Geometry check sheet. Reference: the model listing, model coordinates, mm. Face numbers are marked on the shaded views. Give positions to 0.01 mm unless a question says otherwise; leave off trailing zeros. Write each loop counter-clockwise with the first axis right and the second up, starting at its lowest first coordinate (ties: lowest second). Pieces come first, ordered by that corner, then holes. Notation, with made-up numbers: (32.25, 34) -> (84.25, 34) arc R21 ccw to (84.25, 47) -> close; hole circle Ø1 at (-36, -3). An arc over 180 degrees is marked (long way). One line per item, written item: value.
from build123d import *

# Parameters (mm, degrees)
SKETCH1_W     = 490
SKETCH1_H     = 390
FRAME_DEPTH   = 40
OPENING_START = -1
SKETCH2_W     = 450
SKETCH2_H     = 350
OPENING_DEPTH = 42
PIVOT_0_START = -1
SKETCH3_R     = 3.3
PIVOT_0_DEPTH = 492
PIVOT_1_START = -1
SKETCH4_R     = 3.3
PIVOT_1_DEPTH = 492
PIVOT_2_START = -1
SKETCH5_R     = 3.3
PIVOT_2_DEPTH = 492
PIVOT_3_START = -1
SKETCH6_R     = 3.3
PIVOT_3_DEPTH = 492
PIVOT_4_START = -1
SKETCH7_R     = 3.3
PIVOT_4_DEPTH = 492
PIVOT_5_START = -1
SKETCH8_R     = 3.3
PIVOT_5_DEPTH = 492


with BuildPart() as part:
    # Sketch1 → frame (new body)
    with BuildSketch(Plane(origin=(0, 0, 0), x_dir=(0, 0, -1), z_dir=(1, 0, 0))):
        with Locations((-245, 195)):
            Rectangle(SKETCH1_W, SKETCH1_H)
    extrude(amount=FRAME_DEPTH)


with BuildPart() as body_2:
    # Sketch2 → opening (new body)
    with BuildSketch(Plane(origin=(0, 0, 0), x_dir=(0, 0, -1), z_dir=(1, 0, 0)).offset(OPENING_START)):
        with Locations((-245, 195)):
            Rectangle(SKETCH2_W, SKETCH2_H)
    extrude(amount=OPENING_DEPTH)


with BuildPart() as part_1:
    add(part.part)

    # Combine1: cut body 2
    add(body_2.part, mode=Mode.SUBTRACT)


with BuildPart() as body_2_2:
    # Sketch3 → pivot_0 (new body)
    with BuildSketch(Plane.XY.offset(PIVOT_0_START)):
        with Locations((20, 49.166666667)):
            Circle(SKETCH3_R)
    extrude(amount=PIVOT_0_DEPTH)


with BuildPart() as part_2:
    add(part_1.part)

    # Combine2: cut body 2 2
    add(body_2_2.part, mode=Mode.SUBTRACT)


with BuildPart() as body_2_3:
    # Sketch4 → pivot_1 (new body)
    with BuildSketch(Plane.XY.offset(PIVOT_1_START)):
        with Locations((20, 107.5)):
            Circle(SKETCH4_R)
    extrude(amount=PIVOT_1_DEPTH)


with BuildPart() as part_3:
    add(part_2.part)

    # Combine3: cut body 2 3
    add(body_2_3.part, mode=Mode.SUBTRACT)


with BuildPart() as body_2_4:
    # Sketch5 → pivot_2 (new body)
    with BuildSketch(Plane.XY.offset(PIVOT_2_START)):
        with Locations((20, 165.833333333)):
            Circle(SKETCH5_R)
    extrude(amount=PIVOT_2_DEPTH)


with BuildPart() as part_4:
    add(part_3.part)

    # Combine4: cut body 2 4
    add(body_2_4.part, mode=Mode.SUBTRACT)


with BuildPart() as body_2_5:
    # Sketch6 → pivot_3 (new body)
    with BuildSketch(Plane.XY.offset(PIVOT_3_START)):
        with Locations((20, 224.166666667)):
            Circle(SKETCH6_R)
    extrude(amount=PIVOT_3_DEPTH)


with BuildPart() as part_5:
    add(part_4.part)

    # Combine5: cut body 2 5
    add(body_2_5.part, mode=Mode.SUBTRACT)


with BuildPart() as body_2_6:
    # Sketch7 → pivot_4 (new body)
    with BuildSketch(Plane.XY.offset(PIVOT_4_START)):
        with Locations((20, 282.5)):
            Circle(SKETCH7_R)
    extrude(amount=PIVOT_4_DEPTH)


with BuildPart() as part_6:
    add(part_5.part)

    # Combine6: cut body 2 6
    add(body_2_6.part, mode=Mode.SUBTRACT)


with BuildPart() as body_2_7:
    # Sketch8 → pivot_5 (new body)
    with BuildSketch(Plane.XY.offset(PIVOT_5_START)):
        with Locations((20, 340.833333333)):
            Circle(SKETCH8_R)
    extrude(amount=PIVOT_5_DEPTH)


with BuildPart() as part_7:
    add(part_6.part)

    # Combine7: cut body 2 7
    add(body_2_7.part, mode=Mode.SUBTRACT)


solid = part_7.part
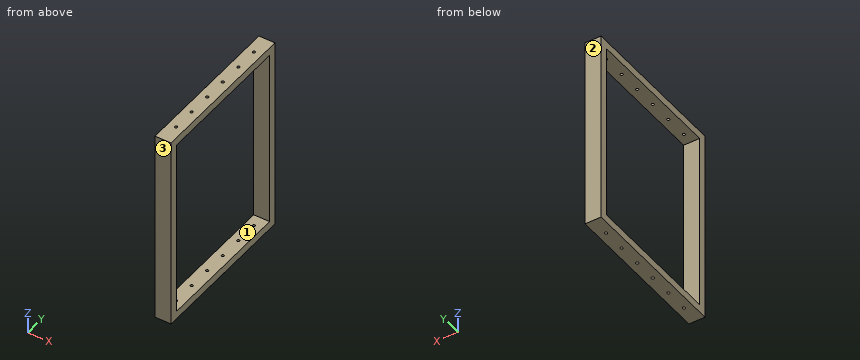
1) Sectioned sample at A-A on z = 236.5. Record the cut outline in (x, y), plus the area to 3 significant figures.
Verdict:
outline: (0, 0) -> (40, 0) -> (40, 20) -> (0, 20) -> close; (0, 370) -> (40, 370) -> (40, 390) -> (0, 390) -> close
area: 1,600 mm^2
2) Sectioned sample at B-B on x = 31.5. Record the cut outline in (y, z), plus the area to 3 significant figures.
Verdict:
outline: (0, 0) -> (390, 0) -> (390, 490) -> (0, 490) -> close; hole (20, 20) -> (370, 20) -> (370, 470) -> (20, 470) -> close
area: 33,600 mm^2
3) Sectioned sample at C-C on y = 62. Record the cut outline in (x, z), plus the area to 3 significant figures.
Verdict:
outline: (0, 0) -> (40, 0) -> (40, 20) -> (0, 20) -> close; (0, 470) -> (40, 470) -> (40, 490) -> (0, 490) -> close
area: 1,600 mm^2
4) Scan lines: probe 1 along Z at (x, y) = (19.5, 302); probe 2 along Y at (x, z) = (9, 102.5); probe 3 along X at (y, z) = (107.5, 484.5). Record each from-to range of solid material in increasing order.
Verdict:
probe 1: 0 to 20, 470 to 490
probe 2: 0 to 20, 370 to 390
probe 3: 0 to 16.7, 23.3 to 40
5) Mould release check, pull along Y, two halves, no side actions. Record for the marked faces 1, 2 and 3: released by +Y, released by -Y, zero draft, split by the parting line, or undercut.
Verdict:
face 1: undercut
face 2: released by +Y
face 3: released by -Y
